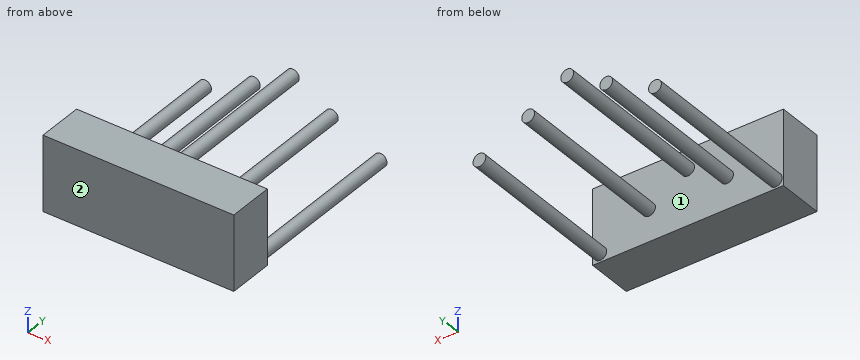
```python
from build123d import *

# Parameters (mm, degrees)
SKETCH1_W           = 79.502
SKETCH1_H           = 31.242
BOSS_EXTRUDE1_DEPTH = 19.05
SKETCH2_R           = 2.667
BOSS_EXTRUDE2_DEPTH = 68.58


with BuildPart() as part:
    # Sketch1 → Boss-Extrude1 (new body)
    with BuildSketch(Plane(origin=(0, 0, 0), x_dir=(1, 0, 0), z_dir=(0, 1, 0))):
        Rectangle(SKETCH1_W, SKETCH1_H)
    extrude(amount=BOSS_EXTRUDE1_DEPTH)

    # Sketch2 → Boss-Extrude2 (add)
    with BuildSketch(Plane(origin=(0, 19.05, 0), x_dir=(1, 0, 0), z_dir=(0, 1, 0))):
        with Locations(Location((-36.576, 12.192, 0), (0, 0, 270))):
            Circle(SKETCH2_R)
        with Locations(Location((-16.256, 2.515131479, 0), (0, 0, 270))):
            Circle(SKETCH2_R)
        with Locations(Location((0, -7.263868521, 0), (0, 0, 270))):
            Circle(SKETCH2_R)
        with Locations(Location((16.256, 2.515131479, 0), (0, 0, 270))):
            Circle(SKETCH2_R)
        with Locations(Location((36.576, 12.192, 0), (0, 0, 270))):
            Circle(SKETCH2_R)
    extrude(amount=BOSS_EXTRUDE2_DEPTH)


solid = part.part
```
Model file for the job. Use its own axes, mm. Face numbers are marked on the shaded views. A direction names the side the tool comes from. Coordinates: 2 decimals unless noted, no trailing zeros. Write each loop counter-clockwise with the first axis right and the second up, starting at its lowest first coordinate (ties: lowest second). Pieces come first, ordered by that corner, then holes. Notation, with made-up numbers: (-38, 56) - (-24, 56) arc R7 cw to (-24, 62) - close; hole circle Ø11 at (19.5, -18). An arc over 180 degrees is marked (long way). Use a Markdown table: item, result. Add a question column.
Item 1: Drop flat-ended pins along their axis: pin 1 (1.5 mm diameter, centred on x = 28.5, z = 4.5, fed in from +Y); pin 2 (1 mm diameter, centred on x = -19, y = 65.5, fed in from -Z); pin 3 (3 mm diameter, centred on y = 41.5, z = 2, fed in from -X); pin 4 (8 mm diameter, centred on x = -22, y = 30.5, fed in from -Z). Give the stop position or say it passes through.
Item 2: Band-saw the part on B-B, the plane y = 56.5. Write the cut outline in (x, z) (3 decimals), and give its area (3 significant figures).
Item 3: Band-saw the part on A-A, the plane x = 0. Write the cut outline in (y, z).
Item 4: Drill centre lines: line 1 along Y through (x, z) = (-23, 5.5); line 2 along X through (y, z) = (23, -10); line 3 along Z through (x, y) = (-16, 52). Where is each one in solid material? Low to high.
Item 5: 3-axis set-ups, long thin cutter, end or side, ignore diameter. For the marked faces 1 and 2: which of +Z, -Z, +X, -X, +Y, -Y reach the whole face in a straight line?
A:
| question | item | result |
|---|---|---|
| 1 | pin 1 | stops at y = 19.05 |
| 1 | pin 2 | stops at z = -3.96 |
| 1 | pin 3 | passes through |
| 1 | pin 4 | stops at z = -4.53 |
| 2 | outline | circle Ø5.334 at (-36.576, -12.192); circle Ø5.334 at (-16.256, -2.515); circle Ø5.334 at (0, 7.264); circle Ø5.334 at (16.256, -2.515); circle Ø5.334 at (36.576, -12.192) |
| 2 | area | 112 mm² |
| 3 | outline | (0, -15.62) - (19.05, -15.62) - (19.05, 4.6) - (87.63, 4.6) - (87.63, 9.93) - (19.05, 9.93) - (19.05, 15.62) - (0, 15.62) - close |
| 4 | line 1 | y = 0 to 19.05 |
| 4 | line 2 | x = -38.1 to -35.06, 35.06 to 38.1 |
| 4 | line 3 | z = -5.17 to 0.14 |
| 5 | face 1 | +Y |
| 5 | face 2 | +Z, -Z, +X, -X, -Y |
